Source: CAD feature listing. Evaluate the final solid. Frame: model axes, mm. Give positions to 0.01 mm unless a question says otherwise; leave off trailing zeros. Order: outer loops, then holes, each group sorted by start corner. A loop starts at its lowest first (then second) coordinate and runs counter-clockwise, first axis right, second up.
from build123d import *

# Parameters (mm, degrees)
CROQUIS1_W              = 1.4
CROQUIS1_H              = 4.5
SALIENTE_EXTRUIR1_DEPTH = 4.65
CROQUIS3_R              = 0.383471958
CORTAR_EXTRUIR1_DEPTH   = 0.25
CROQUIS4_W              = 0.2
CROQUIS4_H              = 0.2
CORTAR_EXTRUIR5_DEPTH   = 0.25
CROQUIS5_W              = 0.51
CROQUIS5_H              = 0.51
SALIENTE_EXTRUIR2_DEPTH = 12.7


with BuildPart() as part:
    # Croquis1 → Saliente-Extruir1 (new body)
    with BuildSketch(Plane(origin=(0, 0, 0), x_dir=(1, 0, 0), z_dir=(0, 1, 0))):
        with Locations((-0.7, -2.25)):
            Rectangle(CROQUIS1_W, CROQUIS1_H)
    extrude(amount=SALIENTE_EXTRUIR1_DEPTH)

    # Croquis3 → Cortar-Extruir1 (cut)
    with BuildSketch(Plane(origin=(0, 4.65, 0), x_dir=(1, 0, 0), z_dir=(0, 1, 0))):
        with Locations(Location((-0.7, -2.25, 0), (0, 0, 270))):
            Circle(CROQUIS3_R)
    extrude(amount=-CORTAR_EXTRUIR1_DEPTH, mode=Mode.SUBTRACT)

    # Croquis4 → Cortar-Extruir5 (cut)
    with BuildSketch(Plane(origin=(0, 4.65, 0), x_dir=(1, 0, 0), z_dir=(0, 1, 0))):
        with Locations((-0.7, -1.75)):
            Rectangle(CROQUIS4_W, CROQUIS4_H)
        with Locations((-0.7, -2.75)):
            Rectangle(CROQUIS4_W, CROQUIS4_H)
    extrude(amount=-CORTAR_EXTRUIR5_DEPTH, mode=Mode.SUBTRACT)

    # Croquis5 → Saliente-Extruir2 (add)
    with BuildSketch(Plane.XZ):
        with Locations((-0.7, 3.5)):
            Rectangle(CROQUIS5_W, CROQUIS5_H)
        with Locations((-0.7, 1.361338898)):
            Rectangle(CROQUIS5_W, CROQUIS5_H)
    extrude(amount=SALIENTE_EXTRUIR2_DEPTH)


solid = part.part
(1) Draft query along Z for faces 1 (the flat face through (-1, 0, 2)), 2 (the flat face through (-1, 4.65, 3)), 3 (the flat face through (-1, 2, 0)), 4 (the flat face through (-1, 2, 4.5)). Return one class per face: +Z half, -Z half, draft (parallel to the pull), parting line (faces both ways), or undercut.
(2) Pin query (flat end, axial travel): pin 1 Ø0.6 at (x, y) = (-0.5, -4.5) entering from +Z (3 decimals); pin 2 Ø0.6 at (y, z) = (-4, 3.5) entering from +X (3 decimals). Return the tip coordinate at first contact, or that it passes through.
(3) Line query: line 1 along X through (y, z) = (4.6, 2.25); line 2 along Z through (x, y) = (-0.6, -2.25) (3 decimals); line 3 along Y through (x, z) = (-0.7, 0.8). Output: solid intervals per line, ascending.
(4) Section C-C, the plane z = 3.5. Return loops of the section in (x, y) (3 decimals).
(5) Section A-A, the plane y = -2. Return loops of the section in (x, z) (3 decimals), plus the area to 3 significant figures.
(6) Section B-B, the plane z = 2.25. Return loops of the section in (x, y).
Checks:
1. face 1: undercut
1. face 2: draft
1. face 3: -Z half
1. face 4: +Z half
2. pin 1: stops at z = 3.755
2. pin 2: stops at x = -0.445
3. line 1: x = -1.4 to -1.08, -0.32 to 0
3. line 2: z = 1.106 to 1.616, 3.245 to 3.755
3. line 3: y = 0 to 4.65
4. outline: (-1.4, 0) - (-0.955, 0) - (-0.955, -12.7) - (-0.445, -12.7) - (-0.445, 0) - (0, 0) - (0, 4.65) - (-1.4, 4.65) - close
5. outline: (-0.955, 1.106) - (-0.445, 1.106) - (-0.445, 1.616) - (-0.955, 1.616) - close; (-0.955, 3.245) - (-0.445, 3.245) - (-0.445, 3.755) - (-0.955, 3.755) - close
5. area: 0.520 mm2
6. outline: (-1.4, 0) - (0, 0) - (0, 4.65) - (-0.32, 4.65) - (-0.32, 4.4) - (-1.08, 4.4) - (-1.08, 4.65) - (-1.4, 4.65) - close
